```python
from build123d import *

# Parameters (mm, degrees)
F0_R     = 11.1
F1_DEPTH = 7
F2_DEPTH = 7
F3_DEPTH = 5


with BuildPart() as f1:
    # F0 (on Front) → F1 (new body)
    with BuildSketch(Plane.XZ):
        with BuildLine():
            ThreePointArc((9.825039, 24.834865), (10.776547, 27.339918), (11.1, 30))
            ThreePointArc((11.1, 30), (-2.660082, 40.776547), (-9.825039, 24.834865))
            ThreePointArc((-9.825039, 24.834865), (0, 18.9), (9.825039, 24.834865))
        make_face()
        with BuildLine():
            ThreePointArc((9.825039, 24.834865), (0, 18.9), (-9.825039, 24.834865))
            ThreePointArc((-9.825039, 24.834865), (-17.166777, 8.96815), (-28.85096, -4.03699))
            ThreePointArc((-28.85096, -4.03699), (-19.293109, -6.023224), (-15.000423, -14.790805))
            ThreePointArc((-15.000423, -14.790805), (-15.360837, -17.596387), (-16.418674, -20.219776))
            ThreePointArc((-16.418674, -20.219776), (-0.060989, -17.733621), (16.209832, -20.736158))
            ThreePointArc((16.209832, -20.736158), (16.251405, -9.649504), (25.865907, -4.128908))
            ThreePointArc((25.865907, -4.128908), (16.086312, 9.378711), (9.825039, 24.834865))
        make_face()
        Circle(F0_R, mode=Mode.SUBTRACT)
        with BuildLine():
            ThreePointArc((-15.000423, -14.790805), (-19.293109, -6.023224), (-28.85096, -4.03699))
            ThreePointArc((-28.85096, -4.03699), (-34.902757, -21.553122), (-16.418674, -20.219776))
            ThreePointArc((-16.418674, -20.219776), (-15.360837, -17.596387), (-15.000423, -14.790805))
        make_face()
        with BuildLine():
            ThreePointArc((36.94726, -15.228892), (33.702735, -7.386602), (25.865907, -4.128908))
            ThreePointArc((25.865907, -4.128908), (16.251405, -9.649504), (16.209832, -20.736158))
            ThreePointArc((16.209832, -20.736158), (28.696343, -25.95702), (36.94726, -15.228892))
        make_face()
    extrude(amount=F1_DEPTH)

    # F0 (on Front) → F2 (join)
    with BuildSketch(Plane.XZ):
        with BuildLine():
            ThreePointArc((9.825039, 24.834865), (10.776547, 27.339918), (11.1, 30))
            ThreePointArc((11.1, 30), (-2.660082, 40.776547), (-9.825039, 24.834865))
            ThreePointArc((-9.825039, 24.834865), (0, 18.9), (9.825039, 24.834865))
        make_face()
        with BuildLine():
            ThreePointArc((9.825039, 24.834865), (0, 18.9), (-9.825039, 24.834865))
            ThreePointArc((-9.825039, 24.834865), (-17.166777, 8.96815), (-28.85096, -4.03699))
            ThreePointArc((-28.85096, -4.03699), (-19.293109, -6.023224), (-15.000423, -14.790805))
            ThreePointArc((-15.000423, -14.790805), (-15.360837, -17.596387), (-16.418674, -20.219776))
            ThreePointArc((-16.418674, -20.219776), (-0.060989, -17.733621), (16.209832, -20.736158))
            ThreePointArc((16.209832, -20.736158), (16.251405, -9.649504), (25.865907, -4.128908))
            ThreePointArc((25.865907, -4.128908), (16.086312, 9.378711), (9.825039, 24.834865))
        make_face()
        Circle(F0_R, mode=Mode.SUBTRACT)
        with BuildLine():
            ThreePointArc((-15.000423, -14.790805), (-19.293109, -6.023224), (-28.85096, -4.03699))
            ThreePointArc((-28.85096, -4.03699), (-34.902757, -21.553122), (-16.418674, -20.219776))
            ThreePointArc((-16.418674, -20.219776), (-15.360837, -17.596387), (-15.000423, -14.790805))
        make_face()
        with BuildLine():
            ThreePointArc((36.94726, -15.228892), (33.702735, -7.386602), (25.865907, -4.128908))
            ThreePointArc((25.865907, -4.128908), (16.251405, -9.649504), (16.209832, -20.736158))
            ThreePointArc((16.209832, -20.736158), (28.696343, -25.95702), (36.94726, -15.228892))
        make_face()
    extrude(amount=F2_DEPTH)

    # F0 (on Front) → F3 (join)
    with BuildSketch(Plane.XZ):
        with BuildLine():
            ThreePointArc((9.825039, 24.834865), (10.776547, 27.339918), (11.1, 30))
            ThreePointArc((11.1, 30), (-2.660082, 40.776547), (-9.825039, 24.834865))
            ThreePointArc((-9.825039, 24.834865), (0, 18.9), (9.825039, 24.834865))
        make_face()
        with BuildLine():
            ThreePointArc((9.825039, 24.834865), (0, 18.9), (-9.825039, 24.834865))
            ThreePointArc((-9.825039, 24.834865), (-17.166777, 8.96815), (-28.85096, -4.03699))
            ThreePointArc((-28.85096, -4.03699), (-19.293109, -6.023224), (-15.000423, -14.790805))
            ThreePointArc((-15.000423, -14.790805), (-15.360837, -17.596387), (-16.418674, -20.219776))
            ThreePointArc((-16.418674, -20.219776), (-0.060989, -17.733621), (16.209832, -20.736158))
            ThreePointArc((16.209832, -20.736158), (16.251405, -9.649504), (25.865907, -4.128908))
            ThreePointArc((25.865907, -4.128908), (16.086312, 9.378711), (9.825039, 24.834865))
        make_face()
        Circle(F0_R, mode=Mode.SUBTRACT)
        with BuildLine():
            ThreePointArc((-15.000423, -14.790805), (-19.293109, -6.023224), (-28.85096, -4.03699))
            ThreePointArc((-28.85096, -4.03699), (-34.902757, -21.553122), (-16.418674, -20.219776))
            ThreePointArc((-16.418674, -20.219776), (-15.360837, -17.596387), (-15.000423, -14.790805))
        make_face()
        with BuildLine():
            ThreePointArc((36.94726, -15.228892), (33.702735, -7.386602), (25.865907, -4.128908))
            ThreePointArc((25.865907, -4.128908), (16.251405, -9.649504), (16.209832, -20.736158))
            ThreePointArc((16.209832, -20.736158), (28.696343, -25.95702), (36.94726, -15.228892))
        make_face()
    extrude(amount=F3_DEPTH)


solid = f1.part
```
Build history of the part. All positions in model axes, mm. Coordinates: 2 decimals unless noted, no trailing zeros. Order: outer loops, then holes, each group sorted by start corner. A loop starts at its lowest first (then second) coordinate and runs counter-clockwise, first axis right, second up. Notation, with made-up numbers: M -33.5,80 L -6.5,80 A3 ccw -6.5,85 Z; hole C -27.75,80.5 d4. An arc over 180 degrees is marked long. One line per question, with ' | ' between items. Start each with the question number.
1. Flat gauge pins, fed straight in: P1, Ø1, axis at y = -6, z = -2.5, coming from the -X side; P2, Ø1.5, axis at x = 12, z = 31.5, coming from the +Y side; P3, Ø1.5, axis at y = -3, z = 33.5, coming from the +X side; P4, Ø4, axis at x = 4.5, y = -5, coming from the +Z side. Where does each tip first touch, or does it go through?
2. Wall check: line 1 along Z through (x, y) = (0, -2.5); line 2 along Z through (x, y) = (-5.5, -0.5); line 3 along X through (y, z) = (-5, 2.5). Give the ranges that are in metal, low to high. Write a range as [from, to].
3. Cut at D-D (x = 28). Write the cut outline in (y, z), plus the area to 3 significant figures.
4. Cut at C-C (y = -6). Write the cut outline in (x, z).
5. Mould opens along Z. For faces 1 (the face through (-9, 0, 8)), 2 (the face through (-35.086, -3.451, -21.307)), 3 (the face through (5.97, -3.45, 9.36)), 4 (the face through (-0.29, -3.45, -17.73)) say: +Z half, -Z half, draft (parallel to the pull), parting line (faces both ways), or undercut.
6. Cut at A-A (z = 0). Write the cut outline in (x, y), plus the area to 3 significant figures.
7. Cut at B-B (x = 0). Write the cut outline in (y, z), plus the area to 3 significant figures.
The answers:
1) P1: stops at x = -27.63 | P2: passes through | P3: stops at x = 10.75 | P4: stops at z = 40.81
2) line 1: z = [-17.73, -11.1], [11.1, 41.1] | line 2: z = [-17.94, -9.64], [9.64, 39.64] | line 3: x = [-22.1, -10.81], [10.81, 20.44]
3) outline: M -7,-26.12 L 0,-26.12 L 0,-4.34 L -7,-4.34 Z | area: 152 mm2
4) outline: M -28.85,-4.04 A11.1 ccw long -16.42,-20.22 A49.87 cw 16.21,-20.74 A11.1 ccw long 25.87,-4.13 A69.15 cw 9.83,24.83 A11.1 ccw 11.1,30 A11.1 ccw long -9.83,24.83 A58.77 cw Z; hole C 0,0 d22.2
5) face 1: draft | face 2: parting line | face 3: undercut | face 4: -Z half
6) outline: M -24.43,-7 L -11.1,-7 L -11.1,0 L -24.43,0 Z; M 11.1,-7 L 22.33,-7 L 22.33,0 L 11.1,0 Z | area: 172 mm2
7) outline: M -7,-17.73 L 0,-17.73 L 0,-11.1 L -7,-11.1 Z; M -7,11.1 L 0,11.1 L 0,41.1 L -7,41.1 Z | area: 256 mm2
